```python
from build123d import *

# Parameters (mm, degrees)
SKETCH_1_R          = 9
EXTRUDE_1_DEPTH     = 2
EXTRUDE_START       = 2
SKETCH_1_3_R        = 2
EXTRUDE_2_DEPTH     = 5
SKETCH_2_R          = 5
SKETCH_2_R_2        = 1.5
EXTRUDE_3_DEPTH     = 0.01
SKETCH_3_R          = 3.5
SKETCH_3_R_2        = 2.6
EXTRUDE_4_DEPTH     = 8
CUT_EXTRUDE_1_REACH = 17.039
SKETCH_2_5_R        = 1.5


with BuildPart() as part:
    # 草图1 → 凸台-拉伸1 (new body)
    with BuildSketch(Plane(origin=(0, 0, 0), x_dir=(0, 0, -1), z_dir=(1, 0, 0))):
        Circle(SKETCH_1_R)
    extrude(amount=EXTRUDE_1_DEPTH)

    # 草图1<3> → 凸台-拉伸2 (add)
    with BuildSketch(Plane(origin=(0, 0, 0), x_dir=(0, 0, -1), z_dir=(1, 0, 0)).offset(EXTRUDE_START)):
        with Locations((0, 6.25)):
            Circle(SKETCH_1_3_R)
        with Locations((-5.412658774, -3.125)):
            Circle(SKETCH_1_3_R)
        with Locations((5.412658774, -3.125)):
            Circle(SKETCH_1_3_R)
    extrude(amount=EXTRUDE_2_DEPTH)

    # 草图2 → 凸台-拉伸3 (add)
    with BuildSketch(Plane.ZY):
        with Locations(Location((0, 0, 0), (0, 0, 180))):
            Circle(SKETCH_2_R)
        with Locations(Location((0, 0, 0), (0, 0, 180))):
            Circle(SKETCH_2_R_2, mode=Mode.SUBTRACT)
    extrude(amount=EXTRUDE_3_DEPTH)

    # 草图3 → 凸台-拉伸4 (add)
    # profile 1 of 5: a face of its own
    with BuildSketch(Plane.ZY.offset(0.01)):
        Circle(SKETCH_3_R)
        Circle(SKETCH_3_R_2, mode=Mode.SUBTRACT)
    # profile 2 of 5: a face of its own
    with BuildSketch(Plane.ZY.offset(0.01)):
        with BuildLine():
            ThreePointArc((-1.204280479, 2.304280479), (-1.838477631, 1.838477631), (-2.304280479, 1.204280479))
            Line((-2.304280479, 1.204280479), (-1.204280479, 1.204280479))
            Line((-1.204280479, 1.204280479), (-1.204280479, 2.304280479))
        make_face()
    # profile 3 of 5: a face of its own
    with BuildSketch(Plane.ZY.offset(0.01)):
        with BuildLine():
            Line((-1.204280479, -1.204280479), (-2.304280479, -1.204280479))
            ThreePointArc((-2.304280479, -1.204280479), (-1.838477631, -1.838477631), (-1.204280479, -2.304280479))
            Line((-1.204280479, -2.304280479), (-1.204280479, -1.204280479))
        make_face()
    # profile 4 of 5: a face of its own
    with BuildSketch(Plane.ZY.offset(0.01)):
        with BuildLine():
            Line((2.304280479, -1.204280479), (1.204280479, -1.204280479))
            Line((1.204280479, -1.204280479), (1.204280479, -2.304280479))
            ThreePointArc((1.204280479, -2.304280479), (1.838477631, -1.838477631), (2.304280479, -1.204280479))
        make_face()
    # profile 5 of 5: a face of its own
    with BuildSketch(Plane.ZY.offset(0.01)):
        with BuildLine():
            Line((1.204280479, 2.304280479), (1.204280479, 1.204280479))
            Line((1.204280479, 1.204280479), (2.304280479, 1.204280479))
            ThreePointArc((2.304280479, 1.204280479), (1.838477631, 1.838477631), (1.204280479, 2.304280479))
        make_face()
    extrude(amount=EXTRUDE_4_DEPTH)

    # 草图2<5> → 切除-拉伸1 (cut, up to next)
    with BuildSketch(Plane.ZY, mode=Mode.PRIVATE) as cut_extrude_1_sk1:
        with Locations(Location((0, 0, 0), (0, 0, 180))):
            Circle(SKETCH_2_5_R)
    cut_extrude_1_tool1 = extrude(cut_extrude_1_sk1.sketch, amount=-CUT_EXTRUDE_1_REACH, mode=Mode.PRIVATE) & part.part
    add(cut_extrude_1_tool1.solids().sort_by_distance((0, 0, 0))[0], mode=Mode.SUBTRACT)


solid = part.part
```
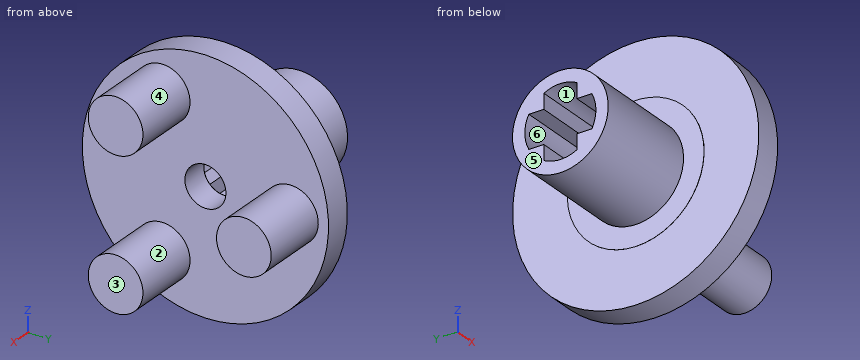
Source: CAD feature listing. Evaluate the final solid. Frame: model axes, mm. Face numbers are marked on the shaded views. A direction names the side the tool comes from. Coordinates: 2 decimals unless noted, no trailing zeros. Loops run counter-clockwise (first coordinate to the right, second up) from the corner with the lowest first, then second, coordinate; pieces in that order, holes last. Notation, with made-up numbers: (11.25, 61.25) -> (37.25, 61.25) arc R15 cw to (37.25, 73.25) -> close; hole circle Ø10 at (24, -1). An arc over 180 degrees is marked (long way). One line per item, written item: value. Start each with the question number.
Q1. Set-up query: the marked faces 1, 2 and 3. Return all of +Z, -Z, +X, -X, +Y, -Y with unobstructed straight access to the full face (end or side cutting, diameter ignored); none if empty.
Q2. Line query: line 1 along Y through (x, z) = (1.2, 0); line 2 along X through (y, z) = (-6, -4.5); line 3 along X through (y, z) = (5.25, -1.5). Output: solid intervals per line, ascending.
Q3. Section query C-C, the plane x = 0.25. Return the cut outline in (y, z), and give its area (3 significant figures).
Q4. Mould query, pull axis Y, two halves, no side actions, for the marked faces 4, 5 and 6. Classes: pulls with the +Y half, pulls with the -Y half, needs draft (parallel to the pull), parting line crosses it, or undercut.
Q5. Contact query for flat-ended pins moving along their axis: P1, Ø1.2, axis at x = -4, y = 2, coming from the +Z side; P2, Ø0.9, axis at x = -4, y = 2, coming from the -Z side; P3, Ø1, axis at y = -4, z = 2.5, coming from the -X side. Output: stop coordinate, or through.
Q6. Section query D-D, the plane z = -6. Return the cut outline in (x, y).
Results:
1. face 1: -X
1. face 2: +X
1. face 3: +Z, -Z, +X, +Y, -Y
2. line 1: -9 to -1.5, 1.5 to 9
2. line 2: 0 to 2
2. line 3: 0 to 7
3. outline: circle Ø18 at (0, 0); hole circle Ø3 at (0, 0)
3. area: 247 mm^2
4. face 4: parting line crosses it
4. face 5: needs draft
4. face 6: undercut
5. P1: z = 3.21
5. P2: z = -3.14
5. P3: x = -0.01
6. outline: (0, -6.71) -> (2, -6.71) -> (2, -5.04) -> (7, -5.04) -> (7, -1.21) -> (2, -1.21) -> (2, 6.71) -> (0, 6.71) -> close
